CAD build for the part. Positions are in the model's coordinates, mm. A direction names the side the tool comes from. Coordinates: 2 decimals unless noted, no trailing zeros. Write each loop counter-clockwise with the first axis right and the second up, starting at its lowest first coordinate (ties: lowest second). Pieces come first, ordered by that corner, then holes.
```python
from build123d import *

# Parameters (mm, degrees)
F0_W     = 127
F0_H     = 130.175
F1_DEPTH = 33.3375
F2_T     = -6.35
F3_W     = 74.93
F3_H     = 26.9875
F4_DEPTH = 35.052
F5_W     = 12.7
F5_H     = 8.6501294995
F5_W_2   = 6.35
F6_DEPTH = 25.4
F7_R     = 5.08
F5_H_2   = 22.5425
F8_DEPTH = 25.4


with BuildPart() as f1:
    # F0 (on Top) → F1 (new body)
    with BuildSketch(Plane.XY):
        with Locations((-63.5, -65.0875)):
            Rectangle(F0_W, F0_H)
    extrude(amount=F1_DEPTH)

    # F2
    f2_openings = [f1.faces().sort_by_distance(p)[0] for p in [
        (-63.5, -65.0875, 0),
    ]]
    offset(amount=F2_T, openings=f2_openings)

    # F3 (on face) → F4 (cut)
    with BuildSketch(Plane(origin=(0, 0, 0), x_dir=(1, 0, 0), z_dir=(0, 0, -1))):
        with Locations((-83.185, 78.58125)):
            Rectangle(F3_W, F3_H)
    extrude(amount=-F4_DEPTH, mode=Mode.SUBTRACT)

    # F5 (on face) → F6 (cut)
    with BuildSketch(Plane.YZ):
        with Locations((-49.2125, -4.3250647498)):
            Rectangle(F5_W, F5_H)
        with Locations((-20.6375, -4.3250647498)):
            Rectangle(F5_W_2, F5_H)
    extrude(amount=-F6_DEPTH, mode=Mode.SUBTRACT)

    # F7
    f7_edges = [f1.edges().sort_by_distance(p)[0] for p in [
        (-127, 0, 16.66875),
        (-127, -130.175, 16.66875),
        (0, -130.175, 16.66875),
        (0, 0, 16.66875),
    ]]
    fillet(f7_edges, radius=F7_R)

    # F5 (on face) → F8 (cut)
    with BuildSketch(Plane.YZ):
        with Locations((-49.2125, 11.27125)):
            Rectangle(F5_W, F5_H_2)
        with Locations((-20.6375, 11.27125)):
            Rectangle(F5_W_2, F5_H_2)
    extrude(amount=-F8_DEPTH, mode=Mode.SUBTRACT)


solid = f1.part
```
Item 1: Two-plate mould, pull along Y, no slides. Class faces 6 (the cylindrical face through (-125.55, -128.65, 16.9)), 7 (the cylindrical face through (-1.449, -1.528, 16.902)), 8 (the flat face through (-64, -123.825, 13)): +Y half, -Y half, draft (parallel to the pull), parting line (faces both ways), or undercut.
Item 2: Flat gauge pins, fed straight in: pin 1 Ø1.9 at (x, z) = (-1.5, 7) entering from -Y; pin 2 Ø1.9 at (x, z) = (-4.5, 13.5) entering from +Y; pin 3 Ø1.5 at (x, y) = (-46, -97.5) entering from -Z; pin 4 Ø3 at (x, y) = (-4, -51) entering from -Z. Where does each tip first touch, or does it go through?
Item 3: Saw through at C-C, the plane y = -58.5. Write the cut outline in (x, z).
Item 4: Which spindle directions (+Z, -Z, +X, -X, +Y, -Y) get a long thin tool onto all of the face, cutting with end or side? Do faces 1 (the flat face through (-6.35, -66, 13)), 2 (the flat face through (-64, -130.175, 16)), 3 (the flat face through (-64, 0, 16)), 4 (the flat face through (-3, -55.562, 11)), 5 (the flat face through (-45.72, -78, 30)). Say none if no direction does.
Item 5: Wall check: line 1 along Y through (x, z) = (-56.5, 8.5) (3 decimals); line 2 along X through (y, z) = (-71.5, 10.5). Give the ranges that are in metal, low to high.
Working result:
1. face 6: -Y half
1. face 7: +Y half
1. face 8: undercut
2. pin 1: stops at y = -129.44
2. pin 2: stops at y = 0
2. pin 3: stops at z = 26.99
2. pin 4: stops at z = 22.54
3. outline: (-127, 0) - (-120.65, 0) - (-120.65, 26.99) - (-6.35, 26.99) - (-6.35, 0) - (0, 0) - (0, 33.34) - (-127, 33.34) - close
4. face 1: -Z
4. face 2: +Z, -Z, +X, -X, -Y
4. face 3: +Z, -Z, +X, -X, +Y
4. face 4: -Z, +X
4. face 5: +Z, -Z
5. line 1: y = -130.175 to -123.825, -6.35 to 0
5. line 2: x = -127 to -120.65, -6.35 to 0
